Geometry: final body of the model. Coordinates: model frame, mm. Give positions to 0.01 mm unless a question says otherwise; leave off trailing zeros. Write each loop counter-clockwise with the first axis right and the second up, starting at its lowest first coordinate (ties: lowest second). Pieces come first, ordered by that corner, then holes. Notation, with made-up numbers: (42.5, -4.5) -> (77.5, -4.5) arc R16 cw to (77.5, 2.5) -> close; hole circle Ø6 at (66.25, -10.5). An arc over 180 degrees is marked (long way). Answer in a Markdown table with one row per item. Add a question column.
Item 1: Material intervals for probe 1 along X at (y, z) = (2.65, 0); probe 2 along Z at (x, y) = (-1.25, 0.6); probe 3 along Z at (x, y) = (-1.25, 2.75), sorted ascending. Write a range as from..to.
Item 2: Section query D-D on z = -17. Output: boundary loops of the cut face in (x, y).
Item 3: Section query C-C on y = 2.1. Output: boundary loops of the cut face in (x, z).
Item 4: Section query A-A on x = 0. Output: boundary loops of the cut face in (y, z), plus the area to 3 significant figures.
Item 5: First-contact query: P1, Ø6, axis at x = 0, z = -37, coming from the -Y side; P2, Ø1, axis at x = 1, y = 3, coming from the -Z side; P3, Ø2, axis at y = 1.5, z = -16.5, coming from the +X side; P4, Ø1, axis at x = -2.5, y = 0.5, coming from the -Z side. Flat tips, straight axial feed; report the tip coordinate or a pass-through.
Item 6: Section query B-B on z = 50. Output: boundary loops of the cut face in (x, y), plus the area to 3 significant figures.
```python
from build123d import *

# Parameters (mm, degrees)
EXTRUDE_1_DEPTH     = 4
SKETCH_2_R          = 2.55
CUT_EXTRUDE_1_DEPTH = 56.3714728
CHAMFER_1_SIZE      = 1


with BuildPart() as part:
    # 草图1 → 凸台-拉伸1 (new body)
    with BuildSketch(Plane(origin=(0, 0, 0), x_dir=(1, 0, 0), z_dir=(0, 1, 0))):
        with BuildLine():
            Line((-4, 47), (-4, 3))
            ThreePointArc((-4, 3), (-5, 0), (-4, -3))
            Line((-4, -3), (-4, -47))
            ThreePointArc((-4, -47), (0, -55), (4, -47))
            Line((4, -47), (4, -3))
            ThreePointArc((4, -3), (5, 0), (4, 3))
            Line((4, 3), (4, 47))
            ThreePointArc((4, 47), (0, 55), (-4, 47))
        make_face()
    extrude(amount=EXTRUDE_1_DEPTH)

    # 草图2 → 切除-拉伸1 (cut, through all)
    with BuildSketch(Plane(origin=(0, 4, 0), x_dir=(1, 0, 0), z_dir=(0, 1, 0))):
        with Locations(Location((0, 50, 0), (0, 0, 270))):
            Circle(SKETCH_2_R)
        with Locations(Location((0, -50, 0), (0, 0, 90))):
            Circle(SKETCH_2_R)
        with Locations(Location((0, 0, 0), (0, 0, 270))):
            Circle(SKETCH_2_R)
    extrude(amount=-CUT_EXTRUDE_1_DEPTH, mode=Mode.SUBTRACT)

    # 倒角1
    chamfer_1_edges = [part.edges().sort_by_distance(p)[0] for p in [
        (4, 0, 25),
        (0, 0, 55),
        (-4, 0, 25),
        (-5, 0, 0),
        (0, 4, 55),
        (4, 4, 25),
        (5, 4, 0),
        (4, 4, -25),
        (0, 4, -55),
        (-4, 4, -25),
        (-5, 4, 0),
        (-4, 0, -25),
        (-4, 4, 25),
        (0, 0, -55),
        (4, 0, -25),
        (5, 0, 0),
    ]]
    chamfer(chamfer_1_edges, length=CHAMFER_1_SIZE)


solid = part.part
```
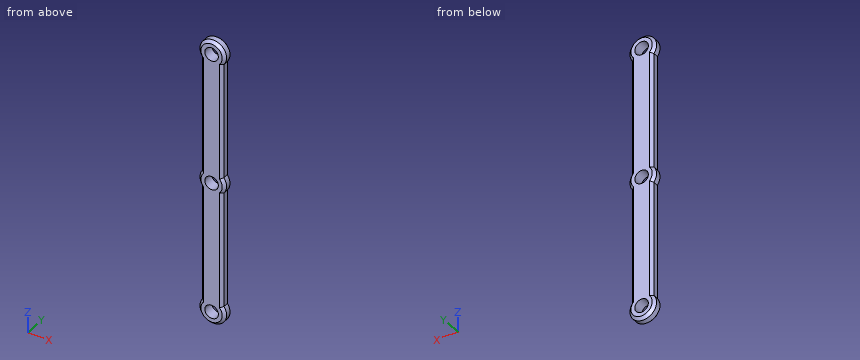
Findings below:
| question | item | result |
|---|---|---|
| 1 | probe 1 | x = -5..-2.55, 2.55..5 |
| 1 | probe 2 | z = -54.43..-52.22, -47.78..-2.22, 2.22..47.78, 52.22..54.43 |
| 1 | probe 3 | z = -54.84..-52.22, -47.78..-2.22, 2.22..47.78, 52.22..54.84 |
| 2 | outline | (-4, 1) -> (-3, 0) -> (3, 0) -> (4, 1) -> (4, 3) -> (3, 4) -> (-3, 4) -> (-4, 3) -> close |
| 3 | outline | (-4, -47) arc R5 ccw (long way) to (4, -47) -> (4, -3) arc R5 ccw to (4, 3) -> (4, 47) arc R5 ccw (long way) to (-4, 47) -> (-4, 3) arc R5 ccw to (-4, -3) -> close; hole circle Ø5.1 at (0, -50); hole circle Ø5.1 at (0, 0); hole circle Ø5.1 at (0, 50) |
| 4 | outline | (0, -54) -> (1, -55) -> (3, -55) -> (4, -54) -> (4, -52.55) -> (0, -52.55) -> close; (0, -47.45) -> (4, -47.45) -> (4, -2.55) -> (0, -2.55) -> close; (0, 2.55) -> (4, 2.55) -> (4, 47.45) -> (0, 47.45) -> close; (0, 52.55) -> (4, 52.55) -> (4, 54) -> (3, 55) -> (1, 55) -> (0, 54) -> close |
| 4 | area | 377 mm^2 |
| 5 | P1 | stops at y = 0 |
| 5 | P2 | stops at z = -54.97 |
| 5 | P3 | stops at x = 4 |
| 5 | P4 | stops at z = -54.39 |
| 6 | outline | (-5, 1) -> (-4, 0) -> (-2.55, 0) -> (-2.55, 4) -> (-4, 4) -> (-5, 3) -> close; (2.55, 0) -> (4, 0) -> (5, 1) -> (5, 3) -> (4, 4) -> (2.55, 4) -> close |
| 6 | area | 17.6 mm^2 |
